```python
from build123d import *

# Parameters (mm, degrees)
SKETCH1_W           = 125
SKETCH1_H           = 180
BASE_EXTRUDE_DEPTH  = 25
SKETCH2_W           = 75
SKETCH2_H           = 120
BOSS_EXTRUDE1_DEPTH = 25
FILLET2_R           = 7.5
FILLET4_R           = 5
SKETCH4_W           = 75
SKETCH4_H           = 57.5
BOSS_EXTRUDE2_DEPTH = 25
SKETCH7_R           = 20
CUT_EXTRUDE2_DEPTH  = 105
SKETCH8_W           = 13
SKETCH8_H           = 57.5
BOSS_EXTRUDE4_DEPTH = 25
SKETCH9_R           = 8
CUT_EXTRUDE3_DEPTH  = 80


with BuildPart() as part:
    # Sketch1 → Base-Extrude (new body)
    with BuildSketch(Plane.XY):
        with Locations((-7.794747082, 12.712840467)):
            Rectangle(SKETCH1_W, SKETCH1_H)
    extrude(amount=BASE_EXTRUDE_DEPTH)

    # Sketch2 → Boss-Extrude1 (add)
    with BuildSketch(Plane.XY.offset(25)):
        with Locations((-7.794747082, 42.712840467)):
            Rectangle(SKETCH2_W, SKETCH2_H)
    extrude(amount=BOSS_EXTRUDE1_DEPTH)

    # Fillet2
    fillet2_edges = [part.edges().sort_by_distance(p)[0] for p in [
        (-45.294747082, 42.712840467, 25),
        (-7.794747082, -17.287159533, 25),
        (29.705252918, 42.712840467, 25),
    ]]
    fillet(fillet2_edges, radius=FILLET2_R)

    # Fillet4
    fillet4_edges = [part.edges().sort_by_distance(p)[0] for p in [
        (54.705252918, 12.712840467, 25),
        (-61.544747082, 102.712840467, 25),
        (-45.294747082, 102.712840467, 41.25),
        (29.705252918, 102.712840467, 41.25),
        (31.901952059, 102.712840467, 27.196699141),
        (-47.491446223, 102.712840467, 27.196699141),
        (-70.294747082, 12.712840467, 25),
        (-7.794747082, -77.287159533, 25),
    ]]
    fillet(fillet4_edges, radius=FILLET4_R)

    # Sketch4 → Boss-Extrude2 (add)
    with BuildSketch(Plane.XY.offset(50)):
        with Locations((-7.794747082, 68.962840467)):
            Rectangle(SKETCH4_W, SKETCH4_H)
    extrude(amount=BOSS_EXTRUDE2_DEPTH)

    # Sketch7 → Cut-Extrude2 (cut)
    with BuildSketch(Plane.XY.offset(75)):
        with Locations((-7.794747082, 67.712840467)):
            Circle(SKETCH7_R)
    extrude(amount=-CUT_EXTRUDE2_DEPTH, mode=Mode.SUBTRACT)

    # Sketch8 → Boss-Extrude4 (add)
    with BuildSketch(Plane.XY.offset(50)):
        with Locations((11.592907965, 11.462840467)):
            Rectangle(SKETCH8_W, SKETCH8_H)
        with Locations((-26.407092035, 11.462840467)):
            Rectangle(SKETCH8_W, SKETCH8_H)
    extrude(amount=BOSS_EXTRUDE4_DEPTH)

    # Sketch9 → Cut-Extrude3 (cut)
    with BuildSketch(Plane.ZY.offset(32.907092035)):
        with Locations((62.5, 11.462840467)):
            Circle(SKETCH9_R)
    extrude(amount=-CUT_EXTRUDE3_DEPTH, mode=Mode.SUBTRACT)


solid = part.part
```
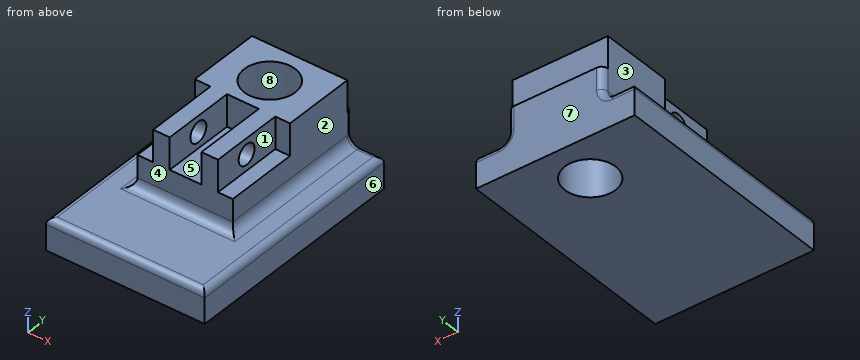
Work out the finished part from the listing and answer in its coordinate system (mm). Face numbers are marked on the shaded views. A direction names the side the tool comes from. Coordinates: 2 decimals unless noted, no trailing zeros. Write each loop counter-clockwise with the first axis right and the second up, starting at its lowest first coordinate (ties: lowest second). Pieces come first, ordered by that corner, then holes.
Q1. A cutting plane is placed at B-B, the plane z = 62.5. Give the vertices of the cut face in (x, y), then the cut area to 3 significant figures.
Q2. Find the intervals of material crossed by line 1 (Y direction, x = 9.75, z = 62.5); line 2 (Z direction, x = 17, y = -34); line 3 (Z direction, x = 24, y = 28), in increasing order.
Q3. Each of these flat-tipped pins is pushed along its axis until it touches: pin 1 Ø4 at (x, y) = (2.5, 100.5) entering from +Z; pin 2 Ø5 at (y, z) = (-12.5, 53.5) entering from +X; pin 3 Ø6 at (x, z) = (-38.5, 58) entering from -Y. Where does it stop, or does it pass through?
Q4. Determine the mould class of the marked faces 6, 7 and 8 for opening direction Y: released by +Y, released by -Y, zero draft, split by the parting line, or undercut.
Q5. A cutting plane is placed at D-D, the plane y = -15. Give the vertices of the cut face in (x, z), then the cut area to 3 significant figures.
Q6. Which of the six approach directions +Z, -Z, +X, -X, +Y, -Y give full straight-line access (tool end or side, diameter ignored) to the marked faces 1, 2, 3, 4 and 5?
Q7. A cutting plane is placed at A-A, the plane x = -24. Give the vertices of the cut face in (y, z).
Q8. A cutting plane is placed at C-C, the plane y = 70.5. Give the vertices of the cut face in (x, z), then the cut area to 3 significant figures.
Findings below:
1. outline: (-45.29, 40.21) - (-32.91, 40.21) - (-32.91, 19.46) - (-19.91, 19.46) - (-19.91, 40.21) - (5.09, 40.21) - (5.09, 19.46) - (18.09, 19.46) - (18.09, 40.21) - (29.71, 40.21) - (29.71, 97.71) - (-45.29, 97.71) - close; (-32.91, -17.29) - (-19.91, -17.29) - (-19.91, 3.46) - (-32.91, 3.46) - close; (5.09, -17.29) - (18.09, -17.29) - (18.09, 3.46) - (5.09, 3.46) - close; hole circle Ø40 at (-7.79, 67.71)
1. area: 4,130 mm2
2. line 1: y = -17.29 to 3.46, 19.46 to 58.11, 77.31 to 97.71
2. line 2: z = 0 to 25
2. line 3: z = 0 to 50
3. pin 1: stops at z = 50
3. pin 2: stops at x = 18.09
3. pin 3: stops at y = 40.21
4. face 6: zero draft
4. face 7: released by +Y
4. face 8: undercut
5. outline: (-70.29, 0) - (54.71, 0) - (54.71, 20) arc R5 ccw to (49.71, 25) - (37.21, 25) arc R7.5 cw to (29.71, 32.5) - (29.71, 50) - (18.09, 50) - (18.09, 75) - (5.09, 75) - (5.09, 50) - (-19.91, 50) - (-19.91, 75) - (-32.91, 75) - (-32.91, 50) - (-45.29, 50) - (-45.29, 32.5) arc R7.5 cw to (-52.79, 25) - (-65.29, 25) arc R5 ccw to (-70.29, 20) - close
5. area: 5,660 mm2
6. face 1: +Z, +X, -Y
6. face 2: +Z, +X, +Y, -Y
6. face 3: +Z, -X, +Y, -Y
6. face 4: +Z, +X, -X, -Y
6. face 5: +Z, -Y
7. outline: (-77.29, 0) - (55.99, 0) - (55.99, 75) - (-17.29, 75) - (-17.29, 32.5) arc R7.5 cw to (-24.79, 25) - (-72.29, 25) arc R5 ccw to (-77.29, 20) - close; (79.43, 0) - (102.71, 0) - (102.71, 50) - (97.71, 50) - (97.71, 75) - (79.43, 75) - close; hole circle Ø16 at (11.46, 62.5)
8. outline: (-70.29, 0) - (-27.6, 0) - (-27.6, 75) - (-45.29, 75) - (-45.29, 32.5) arc R7.5 cw to (-52.79, 25) - (-65.29, 25) arc R5 ccw to (-70.29, 20) - close; (12.01, 0) - (54.71, 0) - (54.71, 20) arc R5 ccw to (49.71, 25) - (37.21, 25) arc R7.5 cw to (29.71, 32.5) - (29.71, 75) - (12.01, 75) - close
8. area: 3,920 mm2
